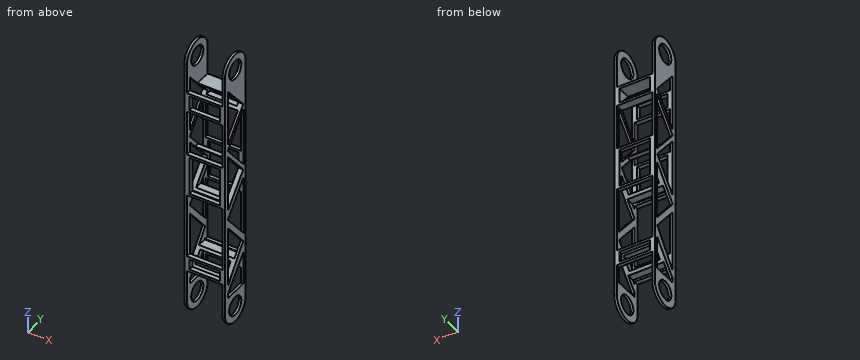
```python
from build123d import *

# Parameters (mm, degrees)
CROQUIS1_R              = 15.25
SALIENTE_EXTRUIR1_DEPTH = 70
CROQUIS2_W              = 57
CROQUIS2_H              = 84.437125565
CROQUIS2_H_2            = 89.497342593
CROQUIS2_H_3            = 103.4811418
CROQUIS2_H_4            = 72.483550253
CORTAR_EXTRUIR1_DEPTH   = 70
CORTAR_EXTRUIR2_DEPTH   = 70
CROQUIS4_R              = 15.25
CORTAR_EXTRUIR3_DEPTH   = 2.5
CROQUIS5_R              = 15.25
CORTAR_EXTRUIR4_DEPTH   = 2.5
CROQUIS6_W              = 49
CROQUIS6_H              = 61.062323931
CORTAR_EXTRUIR5_DEPTH   = 70
CROQUIS7_W              = 49
CROQUIS7_H              = 23.488755438
CORTAR_EXTRUIR6_DEPTH   = 70
CROQUIS8_W              = 49
CROQUIS8_H              = 16.905630738
CORTAR_EXTRUIR7_DEPTH   = 70
CORTAR_EXTRUIR8_DEPTH   = 75


with BuildPart() as part:
    # Croquis1 → Saliente-Extruir1 (new body)
    with BuildSketch(Plane(origin=(0, 0, 0), x_dir=(0, 0, -1), z_dir=(1, 0, 0))):
        with BuildLine():
            Line((-200, 35), (200, 35))
            ThreePointArc((200, 35), (235, 0), (200, -35))
            Line((200, -35), (-200, -35))
            ThreePointArc((-200, -35), (-235, 0), (-200, 35))
        make_face()
        with Locations((-200, 0)):
            Circle(CROQUIS1_R, mode=Mode.SUBTRACT)
        with Locations((200, 0)):
            Circle(CROQUIS1_R, mode=Mode.SUBTRACT)
    extrude(amount=SALIENTE_EXTRUIR1_DEPTH)

    # Croquis2 → Cortar-Extruir1 (cut)
    with BuildSketch(Plane(origin=(0, 35, 0), x_dir=(1, 0, 0), z_dir=(0, 1, 0))):
        with Locations((35, -194.508891983)):
            Rectangle(CROQUIS2_W, CROQUIS2_H)
        with Locations((35, 193.879744257)):
            Rectangle(CROQUIS2_W, CROQUIS2_H_2)
        with Locations((35, 72.484871322)):
            Rectangle(CROQUIS2_W, CROQUIS2_H_3)
        with Locations((35, -84.559798636)):
            Rectangle(CROQUIS2_W, CROQUIS2_H_4)
    extrude(amount=-CORTAR_EXTRUIR1_DEPTH, mode=Mode.SUBTRACT)

    # Croquis3 → Cortar-Extruir2 (cut)
    with BuildSketch(Plane(origin=(70, 0, 0), x_dir=(0, 0, -1), z_dir=(1, 0, 0))):
        with BuildLine():
            Line((-200, -35), (200, -35))
            ThreePointArc((200, -35), (235, 0), (200, 35))
            Line((200, 35), (-200, 35))
            ThreePointArc((-200, 35), (-235, 0), (-200, -35))
        make_face()
        with BuildLine():
            ThreePointArc((-200, 26), (-226, 0), (-200, -26))
            Line((-200, -26), (200, -26))
            ThreePointArc((200, -26), (226, 0), (200, 26))
            Line((200, 26), (-200, 26))
        make_face(mode=Mode.SUBTRACT)
    extrude(amount=-CORTAR_EXTRUIR2_DEPTH, mode=Mode.SUBTRACT)

    # Croquis4 → Cortar-Extruir3 (cut)
    with BuildSketch(Plane(origin=(70, 0, 0), x_dir=(0, 0, -1), z_dir=(1, 0, 0))):
        with BuildLine():
            Line((-200, 26), (200, 26))
            ThreePointArc((200, 26), (226, 0), (200, -26))
            Line((200, -26), (-200, -26))
            ThreePointArc((-200, -26), (-226, 0), (-200, 26))
        make_face()
        with Locations((-200, 0)):
            Circle(CROQUIS4_R, mode=Mode.SUBTRACT)
    extrude(amount=-CORTAR_EXTRUIR3_DEPTH, mode=Mode.SUBTRACT)

    # Croquis5 → Cortar-Extruir4 (cut)
    with BuildSketch(Plane.ZY):
        with BuildLine():
            Line((-200, 26), (200, 26))
            ThreePointArc((200, 26), (226, 0), (200, -26))
            Line((200, -26), (-200, -26))
            ThreePointArc((-200, -26), (-226, 0), (-200, 26))
        make_face()
        with Locations((200, 0)):
            Circle(CROQUIS5_R, mode=Mode.SUBTRACT)
        with Locations((-200, 0)):
            Circle(CROQUIS5_R, mode=Mode.SUBTRACT)
    extrude(amount=-CORTAR_EXTRUIR4_DEPTH, mode=Mode.SUBTRACT)

    # Croquis6 → Cortar-Extruir5 (cut)
    with BuildSketch(Plane(origin=(0, 26, 0), x_dir=(1, 0, 0), z_dir=(0, 1, 0))):
        with Locations((35, -13.786861543)):
            Rectangle(CROQUIS6_W, CROQUIS6_H)
    extrude(amount=-CORTAR_EXTRUIR5_DEPTH, mode=Mode.SUBTRACT)

    # Croquis7 → Cortar-Extruir6 (cut)
    with BuildSketch(Plane(origin=(0, 26, 0), x_dir=(1, 0, 0), z_dir=(0, 1, 0))):
        with Locations((35, -136.545951481)):
            Rectangle(CROQUIS7_W, CROQUIS7_H)
    extrude(amount=-CORTAR_EXTRUIR6_DEPTH, mode=Mode.SUBTRACT)

    # Croquis8 → Cortar-Extruir7 (cut)
    with BuildSketch(Plane(origin=(0, 26, 0), x_dir=(1, 0, 0), z_dir=(0, 1, 0))):
        with Locations((35, 136.678257591)):
            Rectangle(CROQUIS8_W, CROQUIS8_H)
    extrude(amount=-CORTAR_EXTRUIR7_DEPTH, mode=Mode.SUBTRACT)

    # Croquis9 → Cortar-Extruir8 (cut, symmetric)
    with BuildSketch(Plane(origin=(0, 0, 0), x_dir=(0, 0, -1), z_dir=(1, 0, 0))):
        Polygon((-175.016247614, -18.719139012), (-129.175761304, 20.119342374), (-83.252481771, -18.719139012), align=None)
        Polygon((-64.5759486, -18.719139012), (27.853775471, -18.719139012), (-18.361086565, 20.119342374), align=None)
        Polygon((-3.953316698, 20.119342374), (88.969737905, 20.119342374), (42.508210603, -18.719139012), align=None)
        Polygon((175.339862658, 20.119342374), (175.339862658, -18.719139012), (168.473319463, -18.719139012), (122.506063728, 20.119342374), align=None)
        Polygon((-119.659693674, 20.119342374), (-73.771877896, -18.719139012), (-27.662190874, 20.119342374), align=None)
        Polygon((56.100678697, -18.719139012), (102.562205998, 20.119342374), (154.954992104, -18.719139012), align=None)
    extrude(amount=CORTAR_EXTRUIR8_DEPTH, both=True, mode=Mode.SUBTRACT)


solid = part.part
```
Check sheet for the modelled part. Datum: model origin and axes. Units: mm. Round coordinates to 2 decimals unless told otherwise and drop trailing zeros. Order: outer loops, then holes, each group sorted by start corner. A loop starts at its lowest first (then second) coordinate and runs counter-clockwise, first axis right, second up.
1) Section check C-C (z = -78.5). Record the boundary of the cut face in (x, y).
2) Section check A-A (z = -6). Record the boundary of the cut face in (x, y).
3) Section check B-B (x = 54.5). Give the number of separate pieces and of enclosed holes in the cut face, and give its area (3 significant figures).
4) Go/stop test with flat-tipped pins: pin 1 Ø4 at (x, y) = (35.5, 22.5) entering from -Z; pin 2 Ø3 at (x, y) = (50, 14) entering from -Z; pin 3 Ø10 at (x, y) = (23.5, -2.5) entering from +Z; pin 4 Ø1.5 at (x, z) = (42, 118.5) entering from -Y. Record where each tip stops, or that it passes through.
5) Scan lines: line 1 (X direction, y = 12.5, z = 146); line 2 (Y direction, x = 66.6, z = 200); line 3 (Z direction, x = 39, y = -9). Record each from-to range of solid material in increasing order.
Result:
1. outline: (2.5, -26) - (6.5, -26) - (6.5, -18.72) - (2.5, -18.72) - close; (2.5, 0.01) - (6.5, 0.01) - (6.5, 11.37) - (2.5, 11.37) - close; (2.5, 20.12) - (6.5, 20.12) - (6.5, 26) - (2.5, 26) - close; (63.5, -26) - (67.5, -26) - (67.5, -18.72) - (63.5, -18.72) - close; (63.5, 0.01) - (67.5, 0.01) - (67.5, 11.37) - (63.5, 11.37) - close; (63.5, 20.12) - (67.5, 20.12) - (67.5, 26) - (63.5, 26) - close
2. outline: (2.5, -26) - (10.5, -26) - (10.5, -18.72) - (2.5, -18.72) - close; (2.5, -0.35) - (10.5, -0.35) - (10.5, 11.8) - (2.5, 11.8) - close; (2.5, 20.12) - (10.5, 20.12) - (10.5, 26) - (2.5, 26) - close; (59.5, -26) - (67.5, -26) - (67.5, -18.72) - (59.5, -18.72) - close; (59.5, -0.35) - (67.5, -0.35) - (67.5, 11.8) - (59.5, 11.8) - close; (59.5, 20.12) - (67.5, 20.12) - (67.5, 26) - (59.5, 26) - close
3. separate pieces: 16
3. enclosed holes: 0
3. area: 595 mm2
4. pin 1: stops at z = -149.13
4. pin 2: stops at z = -128.23
4. pin 3: stops at z = 152.29
4. pin 4: passes through
5. line 1: x = 2.5 to 10.5, 59.5 to 67.5
5. line 2: y = -26 to -15.25, 15.25 to 26
5. line 3: z = -149.13 to -145.13, -20.74 to -16.74
